Verification items for the finished model (mm, model axes). Face numbers are marked on the shaded views. A direction names the side the tool comes from. Coordinates: 2 decimals unless noted, no trailing zeros. Write each loop counter-clockwise with the first axis right and the second up, starting at its lowest first coordinate (ties: lowest second). Pieces come first, ordered by that corner, then holes. Notation, with made-up numbers: (81.25, 77.25) - (116.25, 77.25) arc R25 cw to (116.25, 89.25) - close; hole circle Ø7 at (67.25, -27). An arc over 180 degrees is marked (long way). Answer as CSV lines item,"result". Start each with the question number.
```python
from build123d import *

# Parameters (mm, degrees)
SKETCH1_R                                          = 1.5875
BOSS_EXTRUDE1_DEPTH                                = 79.375
SKETCH2_W                                          = 19.05
SKETCH2_H                                          = 18.2245
SKETCH2_W_2                                        = 47.625
CUT_EXTRUDE1_DEPTH                                 = 85.302079601
CSK_FOR_10_FLAT_HEAD_MACHINE_SCREW_100_D           = 5.1054
CSK_FOR_10_FLAT_HEAD_MACHINE_SCREW_100_CSINK_D     = 9.779
CSK_FOR_10_FLAT_HEAD_MACHINE_SCREW_100_CSINK_ANGLE = 100
TAP_DRILL_FOR_3_8_16_TAP1_REACH                    = 52.899
TAP_DRILL_FOR_3_8_16_TAP1_BORE_R                   = 3.96875
F_3_8_CLEARANCE_HOLE1_REACH                        = 83.382
F_3_8_CLEARANCE_HOLE1_BORE_R                       = 5.0419


with BuildPart() as part:
    # Sketch1 → Boss-Extrude1 (new body)
    with BuildSketch(Plane(origin=(0, 0, 0), x_dir=(0, 0, -1), z_dir=(1, 0, 0))):
        with BuildLine():
            Line((-12.7, 0), (-12.7, -11.1125))
            Line((-12.7, -11.1125), (12.7, -11.1125))
            Line((12.7, -11.1125), (12.7, 0))
            ThreePointArc((12.7, 0), (0, 12.7), (-12.7, 0))
        make_face()
        with Locations(Location((0, 0, 0), (0, 0, 180))):
            Circle(SKETCH1_R, mode=Mode.SUBTRACT)
    extrude(amount=BOSS_EXTRUDE1_DEPTH)

    # Sketch2 → Cut-Extrude1 (cut, through all)
    with BuildSketch(Plane.XY.offset(12.7)):
        with Locations((15.875, 3.58775)):
            Rectangle(SKETCH2_W, SKETCH2_H)
        with Locations((55.5625, 3.58775)):
            Rectangle(SKETCH2_W_2, SKETCH2_H)
    extrude(amount=-CUT_EXTRUDE1_DEPTH, mode=Mode.SUBTRACT)

    # CSK for _10 Flat Head Machine Screw _100 (through all)
    with Locations(Plane(origin=(0, -5.5245, 0), x_dir=(1, 0, 0), z_dir=(0, 1, 0))):
        with Locations((38.1, 0), (63.5, 0)):
            CounterSinkHole(CSK_FOR_10_FLAT_HEAD_MACHINE_SCREW_100_D / 2, CSK_FOR_10_FLAT_HEAD_MACHINE_SCREW_100_CSINK_D / 2, counter_sink_angle=CSK_FOR_10_FLAT_HEAD_MACHINE_SCREW_100_CSINK_ANGLE)

    # Tap Drill for 3/8-16 Tap1 bore → Tap Drill for 3/8-16 Tap1 (cut, up to next)
    with BuildSketch(Plane(origin=(31.75, 0, 0), x_dir=(0, 0, -1), z_dir=(1, 0, 0)), mode=Mode.PRIVATE) as tap_drill_for_3_8_16_tap1_sk1:
        Circle(TAP_DRILL_FOR_3_8_16_TAP1_BORE_R)
    tap_drill_for_3_8_16_tap1_tool1 = extrude(tap_drill_for_3_8_16_tap1_sk1.sketch, amount=-TAP_DRILL_FOR_3_8_16_TAP1_REACH, mode=Mode.PRIVATE) & part.part
    add(tap_drill_for_3_8_16_tap1_tool1.solids().sort_by_distance((31.75, 0, 0))[0], mode=Mode.SUBTRACT)

    # 3/8 Clearance Hole1 bore → 3/8 Clearance Hole1 (cut, up to next)
    with BuildSketch(Plane.ZY, mode=Mode.PRIVATE) as f_3_8_clearance_hole1_sk1:
        Circle(F_3_8_CLEARANCE_HOLE1_BORE_R)
    f_3_8_clearance_hole1_tool1 = extrude(f_3_8_clearance_hole1_sk1.sketch, amount=-F_3_8_CLEARANCE_HOLE1_REACH, mode=Mode.PRIVATE) & part.part
    add(f_3_8_clearance_hole1_tool1.solids().sort_by_distance((0, 0, 0))[0], mode=Mode.SUBTRACT)


solid = part.part
```
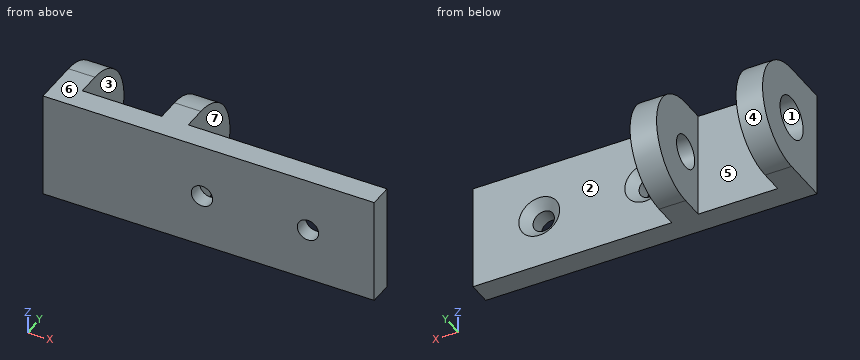
1. Cross-section at C-C (y = 9). Record the cut outline in (x, z).
2. Draft check along X on the marked faces 5, 6 and 7. Enter one of: pulls with the +X half, pulls with the -X half, needs draft (parallel to the pull), parting line crosses it, or undercut.
3. Depth check by flat-ended pin: P1, Ø5.5, axis at y = 7, z = 0.5, coming from the +X side; P2, Ø2, axis at y = 2, z = 4, coming from the -X side; P3, Ø9.5, axis at x = 20.5, z = 5, coming from the +Y side. Enter the tip coordinate at first touch or a pass-through.
4. Scan lines: line 1 along Z through (x, y) = (63.5, -9.25); line 2 along Y through (x, z) = (29.5, 0); line 3 along Y through (x, z) = (39, -11.5). Record each from-to range of solid material in increasing order. Write a range as from..to.
5. Cross-section at A-A (z = 0). Count the separate pieces of the cut face and the enclosed holes in it, and give its area (3 significant figures).
6. Access from +Z, -Z, +X, -X, +Y, -Y to the whole of each face (thin tool, end or side, straight path). Record for the marked faces 1, 2, 3 and 4.
7. Cross-section at B-B (x = 38.1). Record the cut outline in (y, z), and give its area (3 significant figures).
Completed:
1,outline,"(0, -8.96) - (6.35, -8.96) - (6.35, 8.96) - (0, 8.96) - close; (25.4, -8.96) - (31.75, -8.96) - (31.75, 8.96) - (25.4, 8.96) - close"
2,face 5,"undercut"
2,face 6,"needs draft"
2,face 7,"pulls with the +X half"
3,P1,"stops at x = 31.75"
3,P2,"stops at x = 0"
3,P3,"stops at y = -5.52"
4,line 1,"z = -12.7..-2.55, 2.55..12.7"
4,line 2,"y = -11.11..-3.97, 3.97..12.7"
4,line 3,"y = -11.11..-5.52"
5,separate pieces,"5"
5,enclosed holes,"0"
5,area,"494 mm2"
6,face 1,"-X"
6,face 2,"+Z, -Z, +X, +Y"
6,face 3,"+Z, -Z, +Y"
6,face 4,"+X, -X, +Y"
7,outline,"(-11.11, -12.7) - (-5.52, -12.7) - (-5.52, -4.89) - (-7.49, -2.55) - (-11.11, -2.55) - close; (-11.11, 2.55) - (-7.49, 2.55) - (-5.52, 4.89) - (-5.52, 12.7) - (-11.11, 12.7) - close"
7,area,"109 mm2"
